Geometry check sheet. Reference: drawing and pictorial views, mm from the part's lowest x, y, z. Coordinates: 2 decimals unless noted, no trailing zeros. Order: outer loops, then holes, each group sorted by start corner. A loop starts at its lowest first (then second) coordinate and runs counter-clockwise, first axis right, second up. Notation, with made-up numbers: M 17.5,-19 L 60.5,-19 A12 cw 60.5,-1 Z; hole C 4.5,49 d5. An arc over 180 degrees is marked long. Return JSON: item names as keys, results as strings.
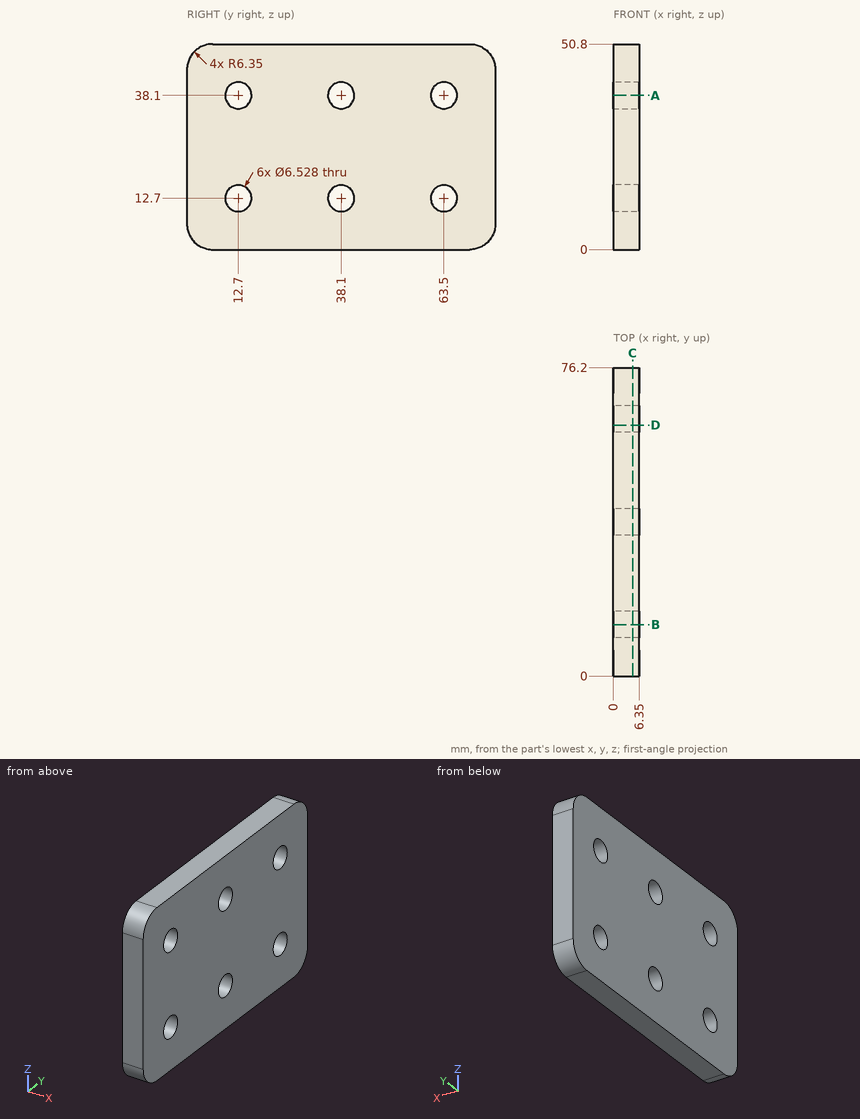
Q1. Cross-section at B-B, the plane y = 12.7. Record the boundary of the cut face in (x, z).
Values:
{"outline": "M 0,0 L 6.35,0 L 6.35,9.44 L 0,9.44 Z; M 0,15.96 L 6.35,15.96 L 6.35,34.84 L 0,34.84 Z; M 0,41.36 L 6.35,41.36 L 6.35,50.8 L 0,50.8 Z"}
Q2. Cross-section at D-D, the plane y = 62. Record the boundary of the cut face in (x, z), and give its area (3 significant figures).
Values:
{"outline": "M 0,0 L 6.35,0 L 6.35,9.8 L 0,9.8 Z; M 0,15.6 L 6.35,15.6 L 6.35,35.2 L 0,35.2 Z; M 0,41 L 6.35,41 L 6.35,50.8 L 0,50.8 Z", "area": "249 mm^2"}
Q3. Cross-section at C-C, the plane x = 4.75. Record the boundary of the cut face in (y, z), and give its area (3 significant figures).
Values:
{"outline": "M 0,6.35 A6.35 ccw 6.35,0 L 69.85,0 A6.35 ccw 76.2,6.35 L 76.2,44.45 A6.35 ccw 69.85,50.8 L 6.35,50.8 A6.35 ccw 0,44.45 Z; hole C 12.7,12.7 d6.53; hole C 12.7,38.1 d6.53; hole C 38.1,12.7 d6.53; hole C 38.1,38.1 d6.53; hole C 63.5,12.7 d6.53; hole C 63.5,38.1 d6.53", "area": "3,640 mm^2"}
Q4. Material ranges on line 1 along Y through (x, z) = (5, 38.1); line 2 along Y through (x, z) = (3.5, 14); line 3 along Z through (x, y) = (4.5, 60.5) (1 decimal), recorded low to high.
Values:
{"line 1": "0 to 9.44, 15.96 to 34.84, 41.36 to 60.24, 66.76 to 76.2", "line 2": "0 to 9.71, 15.69 to 35.11, 41.09 to 60.51, 66.49 to 76.2", "line 3": "0 to 11.4, 14 to 36.8, 39.4 to 50.8"}
Q5. Go/stop test with a flat-tipped pin: pin 1 (5 mm diameter, centred on y = 63.5, z = 12.7, fed in from -X). Record where the tip stops, or that it passes through.
Values:
{"pin 1": "through"}
Q6. Cross-section at A-A, the plane z = 38.1. Record the boundary of the cut face in (x, y).
Values:
{"outline": "M 0,0 L 6.35,0 L 6.35,9.44 L 0,9.44 Z; M 0,15.96 L 6.35,15.96 L 6.35,34.84 L 0,34.84 Z; M 0,41.36 L 6.35,41.36 L 6.35,60.24 L 0,60.24 Z; M 0,66.76 L 6.35,66.76 L 6.35,76.2 L 0,76.2 Z"}
